Build history of the part. All positions in model axes, mm. A direction names the side the tool comes from. Round coordinates to 2 decimals unless told otherwise and drop trailing zeros. Order: outer loops, then holes, each group sorted by start corner. A loop starts at its lowest first (then second) coordinate and runs counter-clockwise, first axis right, second up. Notation, with made-up numbers: (60.25, 26) -> (72.25, 26) arc R17 cw to (72.25, 43) -> close; hole circle Ø7 at (68, 71.5). An arc over 180 degrees is marked (long way). Write item = value, one per line.
from build123d import *
from build123d.topology import SkipClean

# Parameters (mm, degrees)
SKETCH1_R                = 25
SKETCH1_W                = 27.5
SKETCH1_H                = 27.5
BOSS_EXTRUDE1_DEPTH      = 55
BOSS_EXTRUDE2_START      = 5
SKETCH2_R                = 25
SKETCH2_W                = 27.5
SKETCH2_H                = 27.5
BOSS_EXTRUDE2_DEPTH      = 5
SKETCH3_W                = 25
SKETCH3_H                = 50
BOSS_EXTRUDE3_DEPTH      = 80
FILLET1_R                = 2.5
FILLET2_R                = 2.5
SKETCH21_W               = 60
SKETCH21_H               = 20.6
CUT_EXTRUDE1_DEPTH       = 11.3
SKETCH22_W               = 40.5
SKETCH22_H               = 20.6
CUT_EXTRUDE2_DEPTH       = 93.059763198
CUT_EXTRUDE3_DEPTH       = 88.464278423
SKETCH23_R               = 2.15
CUT_EXTRUDE4_DEPTH       = 93.059763198
CUT_EXTRUDE7_DEPTH       = 27.5
CUT_EXTRUDE9_DEPTH       = 93.059763198
CUT_EXTRUDE10_DEPTH      = 91.545224131
CUT_EXTRUDE10_DEPTH_BACK = 91.545224131
SKETCH26_W               = 75.598787472
SKETCH26_H               = 50


with BuildPart() as part:
    # Sketch1 → Boss-Extrude1 (new body)
    with BuildSketch(Plane.XY):
        Circle(SKETCH1_R)
        Rectangle(SKETCH1_W, SKETCH1_H, mode=Mode.SUBTRACT)
    extrude(amount=BOSS_EXTRUDE1_DEPTH)

    # Sketch2 → Boss-Extrude2 (add)
    # profile 1 of 2: a face of its own
    with BuildSketch(Plane(origin=(0, 0, 0), x_dir=(-1, 0, 0), z_dir=(0, 0, -1)).offset(BOSS_EXTRUDE2_START)):
        Circle(SKETCH2_R)
        Rectangle(SKETCH2_W, SKETCH2_H, mode=Mode.SUBTRACT)
    # profile 2 of 2: a face of its own
    with BuildSketch(Plane(origin=(0, 0, 0), x_dir=(-1, 0, 0), z_dir=(0, 0, -1)).offset(BOSS_EXTRUDE2_START)):
        Rectangle(SKETCH2_W, SKETCH2_H)
    extrude(amount=-BOSS_EXTRUDE2_DEPTH)

    # Sketch3 → Boss-Extrude3 (add)
    with BuildSketch(Plane(origin=(0, 0, -5), x_dir=(-1, 0, 0), z_dir=(0, 0, -1))):
        with Locations((12.5, 0)):
            Rectangle(SKETCH3_W, SKETCH3_H)
    extrude(amount=BOSS_EXTRUDE3_DEPTH)

    # Fillet1
    fillet1_edges = [part.edges().sort_by_distance(p)[0] for p in [
        (-13.75, 13.75, 27.5),
        (-13.75, -13.75, 27.5),
        (13.75, -13.75, 27.5),
        (13.75, 13.75, 27.5),
    ]]
    fillet(fillet1_edges, radius=FILLET1_R)

    # Fillet2
    fillet2_edges = [part.edges().sort_by_distance(p)[0] for p in [
        (0, 13.75, 55),
        (-13.75, 0, 55),
        (0, -13.75, 55),
        (13.75, 0, 55),
        (-13.017766953, 13.017766953, 55),
        (-13.017766953, -13.017766953, 55),
        (13.017766953, -13.017766953, 55),
        (13.017766953, 13.017766953, 55),
    ]]
    fillet(fillet2_edges, radius=FILLET2_R)

    # Sketch21 → Cut-Extrude1 (cut)
    with BuildSketch(Plane(origin=(0, 0, 0), x_dir=(0, 0, -1), z_dir=(1, 0, 0))):
        with Locations((52, 0)):
            Rectangle(SKETCH21_W, SKETCH21_H)
    extrude(amount=-CUT_EXTRUDE1_DEPTH, mode=Mode.SUBTRACT)

    # Sketch22 → Cut-Extrude2 (cut, through all)
    with BuildSketch(Plane(origin=(0, 0, 0), x_dir=(0, 0, -1), z_dir=(1, 0, 0))):
        with Locations((51.85, 0)):
            Rectangle(SKETCH22_W, SKETCH22_H)
    extrude(amount=-CUT_EXTRUDE2_DEPTH, mode=Mode.SUBTRACT)

    # Sketch18 → Cut-Extrude3 (cut, through all)
    with BuildSketch(Plane.XY.offset(-5)):
        with BuildLine():
            Line((-25, -25), (0, -25))
            ThreePointArc((0, -25), (-17.67766953, -17.67766953), (-25, 0))
            Line((-25, 0), (-25, -25))
        make_face()
        with BuildLine():
            Line((-25, 25), (-25, 0))
            ThreePointArc((-25, 0), (-17.67766953, 17.67766953), (0, 25))
            Line((0, 25), (-25, 25))
        make_face()
    extrude(amount=-CUT_EXTRUDE3_DEPTH, mode=Mode.SUBTRACT)

    # Sketch23 → Cut-Extrude4 (cut, through all)
    with BuildSketch(Plane(origin=(0, 0, 0), x_dir=(0, 0, -1), z_dir=(1, 0, 0))):
        with Locations(Location((27.85, -5.25, 0), (0, 0, 90))):
            Circle(SKETCH23_R)
        with Locations(Location((75.85, 5.25, 0), (0, 0, 90))):
            Circle(SKETCH23_R)
        with Locations(Location((75.85, -5.25, 0), (0, 0, 90))):
            Circle(SKETCH23_R)
        with Locations(Location((27.85, 5.25, 0), (0, 0, 90))):
            Circle(SKETCH23_R)
    extrude(amount=-CUT_EXTRUDE4_DEPTH, mode=Mode.SUBTRACT)

    # Sketch24 → Cut-Extrude7 (cut, symmetric)
    with BuildSketch(Plane(origin=(0, 0, -51.85), x_dir=(-1, 0, 0), z_dir=(0, 0, -1))):
        with BuildLine():
            Line((22.779596133, 10.3), (13.3, 10.3))
            Line((13.3, 10.3), (13.3, -10.3))
            Line((13.3, -10.3), (22.779596133, -10.3))
            ThreePointArc((22.779596133, -10.3), (25, 0), (22.779596133, 10.3))
        make_face()
    extrude(amount=CUT_EXTRUDE7_DEPTH, both=True, mode=Mode.SUBTRACT)

    # Sketch25 → Cut-Extrude9 (cut, through all)
    with BuildSketch(Plane(origin=(0, 0, 0), x_dir=(0, 0, -1), z_dir=(1, 0, 0))):
        Polygon((85, 25), (20.598787472, 25), (20.598787472, 11.783494563), (83.357288901, 11.783494563), (83.357288901, -11.262677124), (20.598787472, -11.262677124), (20.598787472, -25), (85, -25), (85, -11.262677124), (85, 11.783494563), align=None)
    extrude(amount=-CUT_EXTRUDE9_DEPTH, mode=Mode.SUBTRACT)

    # Sketch26 → Cut-Extrude10 (cut, two sides: drawn at the far end of the back side and taken through both)
    with SkipClean():  # the faces are left unmerged after this step: merging them gives an invalid solid
        with BuildSketch(Plane(origin=(0, 0, 0), x_dir=(0, 0, -1), z_dir=(1, 0, 0)).offset(-CUT_EXTRUDE10_DEPTH_BACK)):
            with Locations((-17.200606264, 0)):
                Rectangle(SKETCH26_W, SKETCH26_H)
        extrude(amount=CUT_EXTRUDE10_DEPTH + CUT_EXTRUDE10_DEPTH_BACK, mode=Mode.SUBTRACT)


solid = part.part
Q1. Probe probe 1 along Z at (x, y) = (-12.6, 5.25); probe 2 along Y at (x, z) = (-14.25, -67.5); probe 3 along Z at (x, y) = (-5, 3). List the from-to ranges inside material, lowest first.
Check values:
probe_1 = -83.36 to -78, -73.7 to -72.1, -31.6 to -30, -25.7 to -20.6
probe_2 = -11.26 to -10.3, 10.3 to 11.78
probe_3 = -83.36 to -82, -22 to -20.6
Q2. Which spindle directions (+Z, -Z, +X, -X, +Y, -Y) get a long thin tool onto all of the face, cutting with end or side? Do faces 4 (the face through (-12, 10.3, -52)), 5 (the face through (-12, 0, -72.1)), 6 (the face through (-13.3, 0, -28)), 7 (the face through (-6, 0, -22)). Say none if no direction does.
Check values:
face_4 = none
face_5 = +X, -X
face_6 = -X
face_7 = +X
Q3. Mould opens along Y. For faces 1 (the face through (-13.3, 0, -76)), 2 (the face through (0, 11, -52)), 3 (the face through (-11, 11.783, -52)) say: released by +Y, released by -Y, zero draft, split by the parting line, or undercut.
Check values:
face_1 = undercut
face_2 = zero draft
face_3 = released by +Y
Q4. Cut at C-C, the plane x = -15.75. List the corners of the cut face in (y, z), and give its area (3 significant figures).
Check values:
outline = (-11.26, -83.36) -> (11.78, -83.36) -> (11.78, -20.6) -> (-11.26, -20.6) -> close; hole (-10.3, -79.35) -> (10.3, -79.35) -> (10.3, -24.35) -> (-10.3, -24.35) -> close
area = 313 mm²
Q5. Cut at B-B, the plane z = -27.85. List the corners of the cut face in (x, y).
Check values:
outline = (-22.78, -10.3) arc R25 ccw to (-22.32, -11.26) -> (0, -11.26) -> (0, -10.3) -> (-11.3, -10.3) -> (-11.3, -7.4) -> (-13.3, -7.4) -> (-13.3, -10.3) -> close; (-22.78, 10.3) -> (-13.3, 10.3) -> (-13.3, 7.4) -> (-11.3, 7.4) -> (-11.3, 10.3) -> (0, 10.3) -> (0, 11.78) -> (-22.05, 11.78) arc R25 ccw to start; (-13.3, -3.1) -> (-11.3, -3.1) -> (-11.3, 3.1) -> (-13.3, 3.1) -> close
Q6. Cut at A-A, the plane y = -1. List the corners of the cut face in (x, z).
Check values:
outline = (-24.98, -83.36) -> (0, -83.36) -> (0, -82) -> (-11.3, -82) -> (-11.3, -72.1) -> (-13.3, -72.1) -> (-13.3, -79.35) -> (-24.98, -79.35) -> close; (-24.98, -24.35) -> (-13.3, -24.35) -> (-13.3, -31.6) -> (-11.3, -31.6) -> (-11.3, -22) -> (0, -22) -> (0, -20.6) -> (-24.98, -20.6) -> close
Q7. Cut at D-D, the plane y = -5. List the corners of the cut face in (x, z), and give its area (3 significant figures).
Check values:
outline = (-24.49, -83.36) -> (0, -83.36) -> (0, -82) -> (-11.3, -82) -> (-11.3, -77.99) -> (-13.3, -77.99) -> (-13.3, -79.35) -> (-24.49, -79.35) -> close; (-24.49, -24.35) -> (-13.3, -24.35) -> (-13.3, -25.71) -> (-11.3, -25.71) -> (-11.3, -22) -> (0, -22) -> (0, -20.6) -> (-24.49, -20.6) -> close; (-13.3, -73.71) -> (-11.3, -73.71) -> (-11.3, -72.1) -> (-13.3, -72.1) -> close; (-13.3, -31.6) -> (-11.3, -31.6) -> (-11.3, -29.99) -> (-13.3, -29.99) -> close
area = 145 mm²
Q8. Flat gauge pins, fed straight in: pin 1 (8 mm diameter, centred on y = 0.5, z = -75, fed in from +X); pin 2 (6 mm diameter, centred on y = -2.5, z = -71, fed in from -X). Where does each tip first touch, or does it go through?
Check values:
pin_1 = -11.3
pin_2 = -13.3
